Geometry check sheet. Reference: the model listing, model coordinates, mm. Face numbers are marked on the shaded views. A direction names the side the tool comes from. Coordinates: 2 decimals unless noted, no trailing zeros. Loops run counter-clockwise (first coordinate to the right, second up) from the corner with the lowest first, then second, coordinate; pieces in that order, holes last. Notation, with made-up numbers: (72.5, -15.5) - (118.5, -15.5) arc R27 ccw to (118.5, 6.5) - close; hole circle Ø4 at (-2.75, 1). An arc over 180 degrees is marked (long way). Write each question's results on one line, items separated by ' | '. Start each with the question number.
(1) Go/stop test with flat-tipped pins: pin 1 Ø4 at (x, y) = (17.71, -17.75) entering from +Z; pin 2 Ø8 at (x, z) = (24.5, 3) entering from +Y; pin 3 Ø2 at (y, z) = (9.5, 12) entering from +X. Record where each tip stops, or that it passes through.
(2) Sectioned sample at A-A (x = 0). Enter the section's corners in (y, z).
(3) Sectioned sample at B-B (y = 0). Enter the section's corners in (x, z).
(4) Material ranges on probe 1 along Y at (x, z) = (0, 11.5); probe 2 along Z at (x, y) = (-32, -7); probe 3 along Y at (x, z) = (2, 6.25), recorded low to high.
(5) Sectioned sample at C-C (y = 25). Enter the section's corners in (x, z).
(6) Access from +Z, -Z, +X, -X, +Y, -Y to the whole of each face (thin tool, end or side, straight path). Record for the marked faces 1 and 2.
(7) Sectioned sample at D-D (z = 8.5). Enter the section's corners in (x, y).
(8) Mould release check, pull along X, two halves, no side actions. Record for the marked faces 3, 4 and 5: pulls with the +X half, pulls with the -X half, needs draft (parallel to the pull), parting line crosses it, or undercut.
from build123d import *

# Parameters (mm, degrees)
SKETCH1_R           = 37.5
BOSS_EXTRUDE1_DEPTH = 2
SKETCH2_R           = 1.5
CUT_EXTRUDE1_DEPTH  = 10
CIRPATTERN1_COUNT   = 8
SKETCH3_R           = 10
SKETCH3_R_2         = 5
BOSS_EXTRUDE2_DEPTH = 12


with BuildPart() as part:
    # Sketch1 → Boss-Extrude1 (new body)
    with BuildSketch(Plane.XY):
        Circle(SKETCH1_R)
    extrude(amount=BOSS_EXTRUDE1_DEPTH)

    # Sketch2 → Cut-Extrude1 (cut)
    with BuildSketch(Plane.XY.offset(2)):
        with Locations((0, 25)):
            Circle(SKETCH2_R)
    cut_extrude1 = extrude(amount=-CUT_EXTRUDE1_DEPTH, mode=Mode.SUBTRACT)

    # CirPattern1: Cut-Extrude1 ×8 about axis
    cirpattern1_axis = Axis((0, -0.040064103, 0), (0, 0, 1))
    for i in range(1, CIRPATTERN1_COUNT):
        add(cut_extrude1.rotate(cirpattern1_axis, i * 360 / CIRPATTERN1_COUNT), mode=Mode.SUBTRACT)

    # Sketch3 → Boss-Extrude2 (add)
    with BuildSketch(Plane.XY.offset(2)):
        Circle(SKETCH3_R)
        Circle(SKETCH3_R_2, mode=Mode.SUBTRACT)
    extrude(amount=BOSS_EXTRUDE2_DEPTH)


solid = part.part
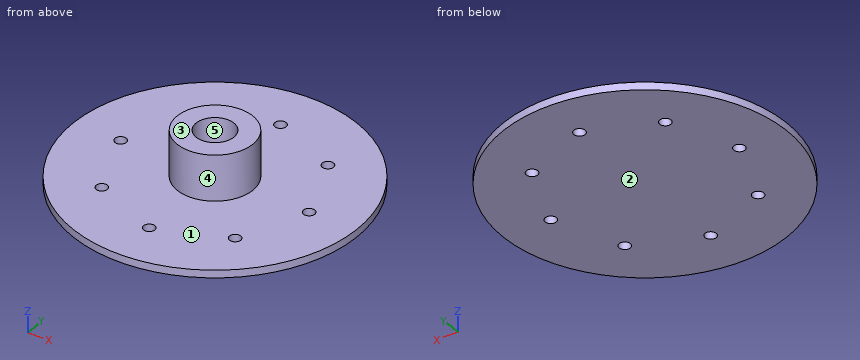
Outcome:
1) pin 1: stops at z = 2 | pin 2: stops at y = 31.32 | pin 3: stops at x = 5.27
2) outline: (-37.5, 0) - (-26.58, 0) - (-26.58, 2) - (-37.5, 2) - close; (-23.58, 0) - (23.5, 0) - (23.5, 2) - (10, 2) - (10, 14) - (5, 14) - (5, 2) - (-5, 2) - (-5, 14) - (-10, 14) - (-10, 2) - (-23.58, 2) - close; (26.5, 0) - (37.5, 0) - (37.5, 2) - (26.5, 2) - close
3) outline: (-37.5, 0) - (-26.54, 0) - (-26.54, 2) - (-37.5, 2) - close; (-23.54, 0) - (23.54, 0) - (23.54, 2) - (10, 2) - (10, 14) - (5, 14) - (5, 2) - (-5, 2) - (-5, 14) - (-10, 14) - (-10, 2) - (-23.54, 2) - close; (26.54, 0) - (37.5, 0) - (37.5, 2) - (26.54, 2) - close
4) probe 1: y = -10 to -5, 5 to 10 | probe 2: z = 0 to 2 | probe 3: y = -9.8 to -4.58, 4.58 to 9.8
5) outline: (-27.95, 0) - (-1.5, 0) - (-1.5, 2) - (-27.95, 2) - close; (1.5, 0) - (27.95, 0) - (27.95, 2) - (1.5, 2) - close
6) face 1: +Z | face 2: -Z, +X, -X, +Y, -Y
7) outline: circle Ø20 at (0, 0); hole circle Ø10 at (0, 0)
8) face 3: needs draft | face 4: parting line crosses it | face 5: undercut
